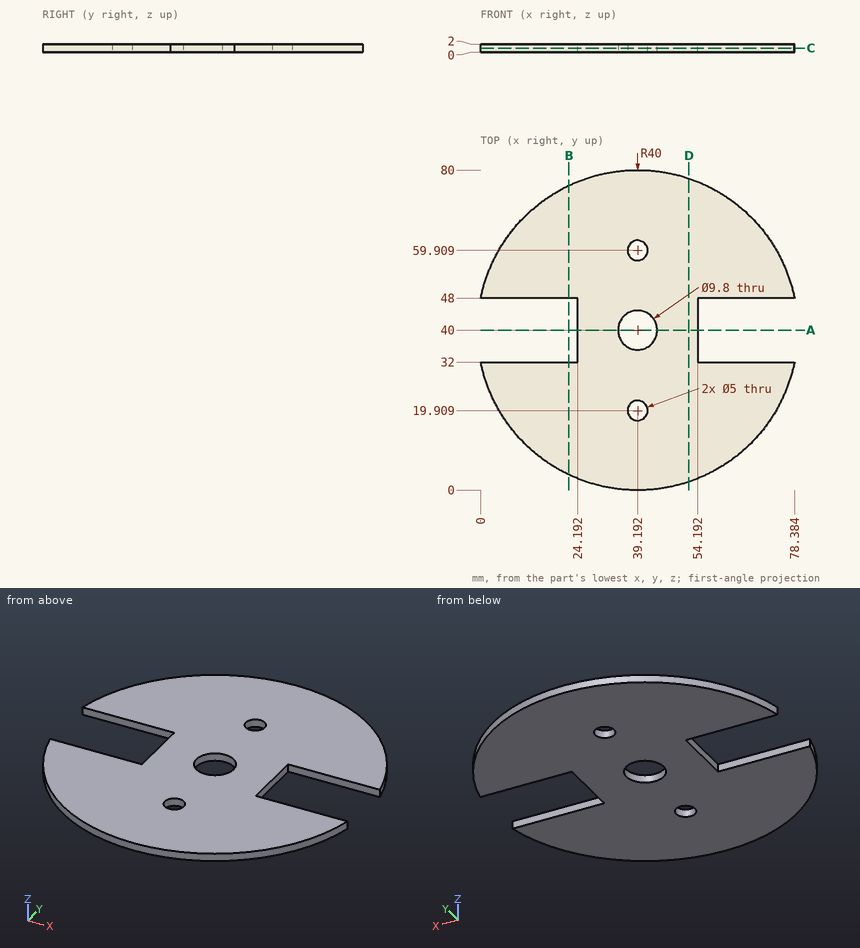
Geometry check sheet. Reference: drawing and pictorial views, mm from the part's lowest x, y, z. Coordinates: 2 decimals unless noted, no trailing zeros. Order: outer loops, then holes, each group sorted by start corner. A loop starts at its lowest first (then second) coordinate and runs counter-clockwise, first axis right, second up. Notation, with made-up numbers: (13, 21.5) - (62, 21.5) arc R6 ccw to (62, 32.5) - close; hole circle Ø6 at (42, -22.5). An arc over 180 degrees is marked (long way). Answer in a Markdown table with one row per item. Add a question column.
1) Gauge pin test, flat ends, axial feed: P1, Ø0.6, axis at y = 39, z = 1.5, coming from the +X side; P2, Ø0.6, axis at x = 64.5, z = 1, coming from the +Y side; P3, Ø4.5, axis at x = 39.19, y = 19.91, coming from the +Z side; P4, Ø0.6, axis at x = 18, z = 1, coming from the -Y side. Record the tip position at first contact, or that the pin passes through.
2) Cross-section at A-A, the plane y = 40. Record the cut outline in (x, z), then the cut area to 3 significant figures.
3) Cross-section at D-D, the plane x = 52. Record the cut outline in (y, z).
4) Cross-section at B-B, the plane x = 22. Record the cut outline in (y, z).
5) Cross-section at C-C, the plane z = 0.95. Record the cut outline in (x, y), then the cut area to 3 significant figures.
6) Material ranges on line 1 along X through (y, z) = (47, 0.5); line 2 along Y through (x, z) = (57, 0.25); line 3 along Y through (x, z) = (9, 1.2), recorded low to high. Write a range as [from, to].
Check result:
| question | item | result |
|---|---|---|
| 1 | P1 | stops at x = 54.19 |
| 1 | P2 | stops at y = 71.22 |
| 1 | P3 | passes through |
| 1 | P4 | stops at y = 5.89 |
| 2 | outline | (24.19, 0) - (34.29, 0) - (34.29, 2) - (24.19, 2) - close; (44.09, 0) - (54.19, 0) - (54.19, 2) - (44.09, 2) - close |
| 2 | area | 40.4 mm² |
| 3 | outline | (2.11, 0) - (77.89, 0) - (77.89, 2) - (2.11, 2) - close |
| 4 | outline | (3.88, 0) - (32, 0) - (32, 2) - (3.88, 2) - close; (48, 0) - (76.12, 0) - (76.12, 2) - (48, 2) - close |
| 5 | outline | (0, 32) arc R40 ccw to (78.38, 32) - (54.19, 32) - (54.19, 48) - (78.38, 48) arc R40 ccw to (0, 48) - (24.19, 48) - (24.19, 32) - close; hole circle Ø9.8 at (39.19, 40); hole circle Ø5 at (39.19, 19.91); hole circle Ø5 at (39.19, 59.91) |
| 5 | area | 4,120 mm² |
| 6 | line 1 | x = [24.19, 54.19] |
| 6 | line 2 | y = [4.18, 32], [48, 75.82] |
| 6 | line 3 | y = [13.76, 32], [48, 66.24] |
